from build123d import *

# Parameters (mm, degrees)
BOX008_W     = 27.5
BOX008_H     = 122.5
BOX008_DEPTH = 0.5
FILLET005_R  = 3
BOX007_W     = 28.5
BOX007_H     = 123.5
BOX007_DEPTH = 0.5
FILLET004_R  = 3.5


with BuildPart() as fillet005:
    # Box008 → Box008 (new body)
    with BuildSketch(Plane(origin=(8, 22, 0), x_dir=(1, 0, 0), z_dir=(0, 0, 1))):
        with Locations((13.75, 61.25)):
            Rectangle(BOX008_W, BOX008_H)
    extrude(amount=BOX008_DEPTH)

    # Fillet005
    fillet005_edges = [fillet005.edges().sort_by_distance(p)[0] for p in [
        (8, 22, 0.25),
        (8, 144.5, 0.25),
        (35.5, 22, 0.25),
        (35.5, 144.5, 0.25),
    ]]
    fillet(fillet005_edges, radius=FILLET005_R)


with BuildPart() as fillet005_1:
    # Fillet005 placement: moved
    add(fillet005.part.moved(Location((0.5, 1, 0))))


with BuildPart() as cut005:
    # Box007 → Box007 (new body)
    with BuildSketch(Plane(origin=(8.5, 22.5, 0), x_dir=(1, 0, 0), z_dir=(0, 0, 1))):
        with Locations((14.25, 61.75)):
            Rectangle(BOX007_W, BOX007_H)
    extrude(amount=BOX007_DEPTH)

    # Fillet004
    fillet004_edges = [cut005.edges().sort_by_distance(p)[0] for p in [
        (8.5, 22.5, 0.25),
        (8.5, 146, 0.25),
        (37, 22.5, 0.25),
        (37, 146, 0.25),
    ]]
    fillet(fillet004_edges, radius=FILLET004_R)


with BuildPart() as cut005_1:
    # Fillet004 placement: moved
    add(cut005.part.moved(Location((-0.5, 0, 0))))

    # Cut005: cut Fillet005
    add(fillet005_1.part, mode=Mode.SUBTRACT)


solid = cut005_1.part
Model file for the job. Use its own axes, mm. A direction names the side the tool comes from. Give positions to 0.01 mm unless a question says otherwise; leave off trailing zeros. Loops run counter-clockwise (first coordinate to the right, second up) from the corner with the lowest first, then second, coordinate; pieces in that order, holes last.
1) Tool access for faces 1 (the cylindrical face through (35.1, 23.86, 0.25)), 2 (the cylindrical face through (35.5, 144.95, 0.25)): list every direction of +Z, -Z, +X, -X, +Y, -Y with a clear straight run to the whole face (end or side of a thin tool).
2) Wall check: line 1 (X direction, y = 46.5, z = 0.1); line 2 (Y direction, x = 15.75, z = 0.1); line 3 (Y direction, x = 34.75, z = 0.2). Give the ranges that are in metal, low to high.
3) Pull direction X, two halves, no side cores. Call faces 3 (the cylindrical face through (35.14, 144.6, 0.25)), 4 (the cylindrical face through (35.45, 23.5, 0.25)), 5 (the cylindrical face through (9, 144.95, 0.25)): +X half, -X half, draft (parallel to the pull), parting line (faces both ways), or undercut.
4) Saw through at A-A (y = 51.5). Write the cut outline in (x, z).
5) Saw through at B-B (z = 0.2). Write the cut outline in (x, y), plus the area to 3 significant figures.
6) Saw through at C-C (x = 21.25). Write the cut outline in (y, z), plus the area to 3 significant figures.
Answer block:
1. face 1: +Z, -Z
1. face 2: +Z, -Z, +X, +Y
2. line 1: x = 8 to 8.5, 36 to 36.5
2. line 2: y = 22.5 to 23, 145.5 to 146
2. line 3: y = 22.97 to 23.56, 144.94 to 145.53
3. face 3: undercut
3. face 4: +X half
3. face 5: -X half
4. outline: (8, 0) - (8.5, 0) - (8.5, 0.5) - (8, 0.5) - close; (36, 0) - (36.5, 0) - (36.5, 0.5) - (36, 0.5) - close
5. outline: (8, 26) arc R3.5 ccw to (11.5, 22.5) - (33, 22.5) arc R3.5 ccw to (36.5, 26) - (36.5, 142.5) arc R3.5 ccw to (33, 146) - (11.5, 146) arc R3.5 ccw to (8, 142.5) - close; hole (8.5, 26) arc R3 ccw to (11.5, 23) - (33, 23) arc R3 ccw to (36, 26) - (36, 142.5) arc R3 ccw to (33, 145.5) - (11.5, 145.5) arc R3 ccw to (8.5, 142.5) - close
5. area: 148 mm2
6. outline: (22.5, 0) - (23, 0) - (23, 0.5) - (22.5, 0.5) - close; (145.5, 0) - (146, 0) - (146, 0.5) - (145.5, 0.5) - close
6. area: 0.500 mm2
